Answer from the drawing. Dimensions are ordinates in mm from the lowest x, y and z of the part. A direction names the side the tool comes from. Round coordinates to 2 decimals unless told otherwise and drop trailing zeros. Order: outer loops, then holes, each group sorted by start corner. A loop starts at its lowest first (then second) coordinate and runs counter-clockwise, first axis right, second up. Notation, with made-up numbers: (0.5, 43.5) -> (17.5, 43.5) arc R13 ccw to (17.5, 67.5) -> close; hole circle Ø10 at (-19, 80). An arc over 180 degrees is marked (long way). Use a Markdown table: item, result. Add a question column.
1. For the marked faces 3 and 4, determine the directions among +Z, -Z, +X, -X, +Y, -Y from which every point of the face is accessible in a straight line to the end or side of a thin tool.
2. Given pin 1 (0.6 mm diameter, centred on x = 12, z = 7.5, fed in from -Y); pin 2 (8 mm diameter, centred on x = 20, y = 15.5, fed in from +Z); pin 3 (8 mm diameter, centred on y = 7.5, z = 10, fed in from -X); pin 4 (1 mm diameter, centred on y = 6, z = 20.5, fed in from +X), each flat-ended and moving along its own axis, determine where each tip first touches the part or whether it passes through.
3. Section D-D, the plane x = 6.75 is taken. Give the vertices of the cut face in (y, z), then the cut area to 3 significant figures.
4. Section B-B, the plane z = 2.25 is taken. Give the vertices of the cut face in (x, y) (1 decimal), then the cut area to 3 significant figures.
5. The mould has two halves that part along X. Classify the marked faces 1 and 2: +X half, -X half, draft (parallel to the pull), parting line (faces both ways), or undercut.
6. Consider L1, parallel to Y at x = 2, z = 17; L2, parallel to X at y = 0.35, z = 7.5 (1 decimal); L3, parallel to X at y = 17.25, z = 3 (1 decimal). Determine where each line is inside the solid, lowest interval first. Write a range as [from, to].
7. Section C-C, the plane y = 4 is taken. Give the vertices of the cut face in (x, z).
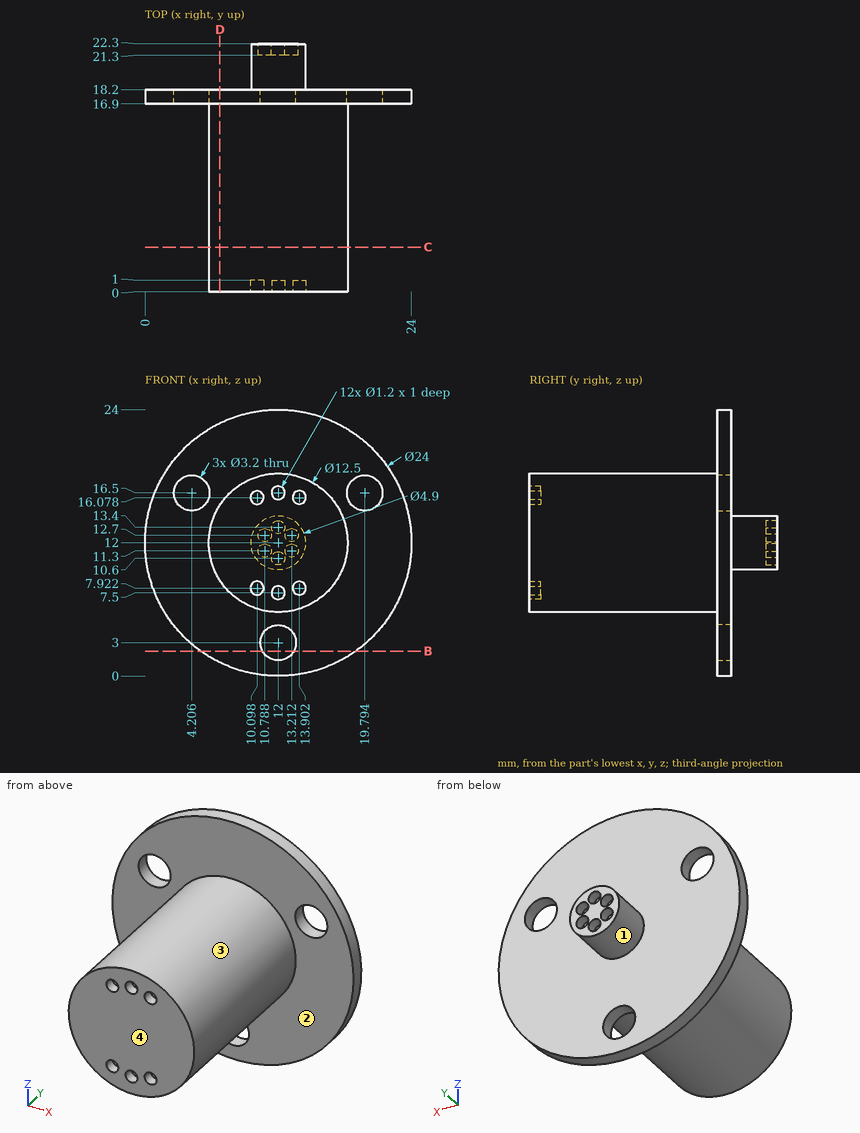
Verdict:
| question | item | result |
|---|---|---|
| 1 | face 3 | -Y |
| 1 | face 4 | +Z, -Z, +X, -X, -Y |
| 2 | pin 1 | stops at y = 1 |
| 2 | pin 2 | stops at z = 23.22 |
| 2 | pin 3 | stops at x = 5.75 |
| 2 | pin 4 | passes through |
| 3 | outline | (0, 8.61) -> (16.9, 8.61) -> (16.9, 1.21) -> (18.2, 1.21) -> (18.2, 22.79) -> (16.9, 22.79) -> (16.9, 15.39) -> (0, 15.39) -> close |
| 3 | area | 143 mm2 |
| 4 | outline | (5, 16.9) -> (10.6, 16.9) -> (10.6, 18.2) -> (5, 18.2) -> close; (13.4, 16.9) -> (19, 16.9) -> (19, 18.2) -> (13.4, 18.2) -> close |
| 4 | area | 14.5 mm2 |
| 5 | face 1 | parting line |
| 5 | face 2 | draft |
| 6 | L1 | y = [16.9, 18.2] |
| 6 | L2 | x = [7.7, 9.7], [10.5, 11.4], [12.6, 13.5], [14.3, 16.3] |
| 6 | L3 | x = [4.1, 10.4], [13.6, 19.9] |
| 7 | outline | circle Ø12.5 at (12, 12) |
